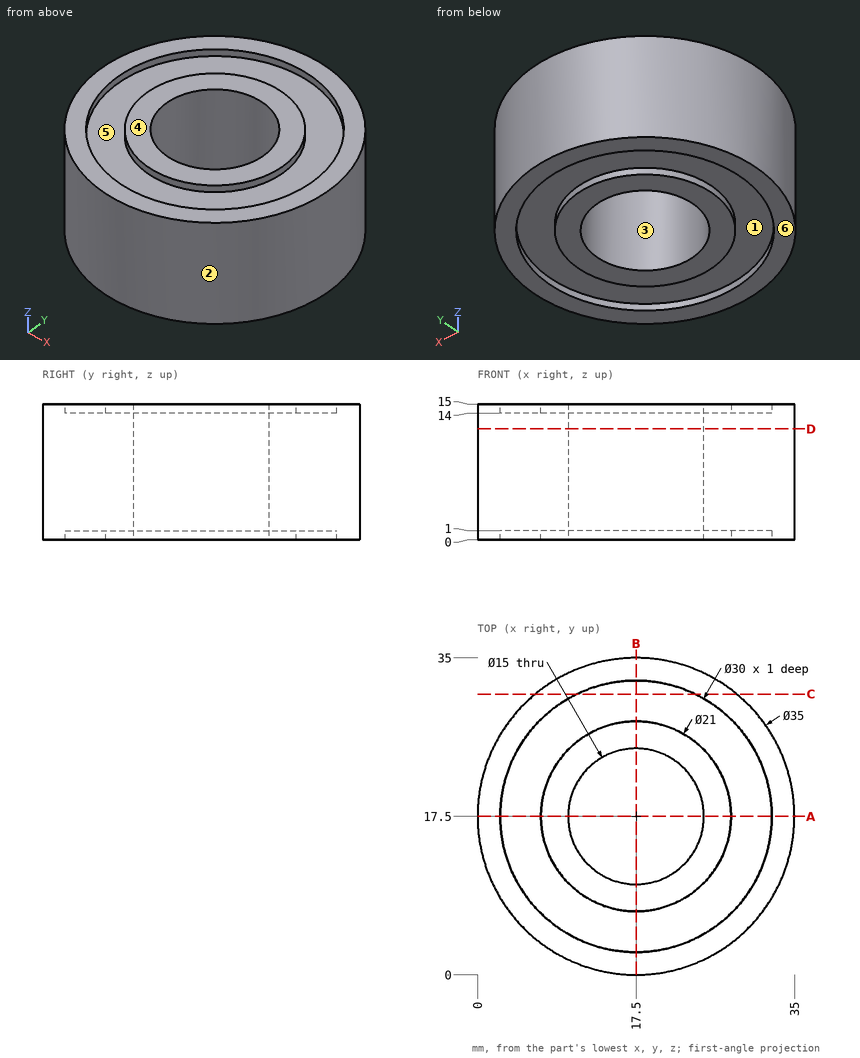
The drawing under review shows one solid part. Ordinate dimensions are in mm from its lowest x, y, z. A direction names the side the tool comes from. Give positions to 0.01 mm unless a question says otherwise; leave off trailing zeros. Order: outer loops, then holes, each group sorted by start corner. A loop starts at its lowest first (then second) coordinate and runs counter-clockwise, first axis right, second up. Notation, with made-up numbers: (-25, 89.5) -> (14, 89.5) arc R7 ccw to (14, 94.5) -> close; hole circle Ø3 at (72, 20.5). An arc over 180 degrees is marked (long way). Write item = value, one per line. Start each with the question number.
(1) For the marked faces 5 and 6, list the 3-axis set-ups (+Z, -Z, +X, -X, +Y, -Y) from which the entire face can be reached by the end or side of a thin tool; tool diameter is ignored.
(2) For pin 1 (2 mm diameter, centred on x = 5.5, z = 3.5, fed in from -Y); pin 2 (6 mm diameter, centred on y = 21.5, z = 12.5, fed in from +X); pin 3 (6 mm diameter, centred on x = 23, z = 2.5, fed in from +Y), all flat-tipped, find the tip position at first contact; note any pin that passes through.
(3) Mouldability with a two-part tool opening along Y and no side actions: class the marked faces 1, 2, 3 and 4 as +Y half, -Y half, draft (parallel to the pull), parting line (faces both ways), or undercut.
(4) To check wall thickness, follow line 1 along Y through (x, z) = (17.5, 14.6); line 2 along Y through (x, z) = (17.5, 11.5); line 3 along Z through (x, y) = (8, 23). State the ranges of each line that lie inside material, in increasing order.
(5) We need section C-C on y = 31. Write out the cut boundary in (x, z).
(6) We need section D-D on z = 12.25. Write out the cut boundary in (x, y), plus the area to 3 significant figures.
(7) We need section A-A on y = 17.5. Write out the cut boundary in (x, z).
Numbers:
q1.face_5 = +Z
q1.face_6 = -Z, +X, -X, +Y, -Y
q2.pin_1 = 3.89
q2.pin_2 = 34.97
q2.pin_3 = 34.82
q3.face_1 = undercut
q3.face_2 = parting line
q3.face_3 = undercut
q3.face_4 = draft
q4.line_1 = 0 to 2.5, 7 to 10, 25 to 28, 32.5 to 35
q4.line_2 = 0 to 10, 25 to 35
q4.line_3 = 1 to 14
q5.outline = (6.36, 0) -> (10.96, 0) -> (10.96, 1) -> (24.04, 1) -> (24.04, 0) -> (28.64, 0) -> (28.64, 15) -> (24.04, 15) -> (24.04, 14) -> (10.96, 14) -> (10.96, 15) -> (6.36, 15) -> close
q6.outline = circle Ø35 at (17.5, 17.5); hole circle Ø15 at (17.5, 17.5)
q6.area = 785 mm^2
q7.outline = (0, 0) -> (2.5, 0) -> (2.5, 1) -> (7, 1) -> (7, 0) -> (10, 0) -> (10, 15) -> (7, 15) -> (7, 14) -> (2.5, 14) -> (2.5, 15) -> (0, 15) -> close; (25, 0) -> (28, 0) -> (28, 1) -> (32.5, 1) -> (32.5, 0) -> (35, 0) -> (35, 15) -> (32.5, 15) -> (32.5, 14) -> (28, 14) -> (28, 15) -> (25, 15) -> close
